from build123d import *

# Parameters (mm, degrees)
SKETCH_1_W      = 450
SKETCH_1_H      = 390
SKETCH_1_R      = 157.5
SKETCH_1_R_2    = 6
SKETCH_1_R_3    = 20
EXTRUDE_1_DEPTH = 24


with BuildPart() as part:
    # 草图1 → 凸台-拉伸1 (new body)
    with BuildSketch(Plane.XY):
        Rectangle(SKETCH_1_W, SKETCH_1_H)
        with Locations((-45, 0)):
            Circle(SKETCH_1_R, mode=Mode.SUBTRACT)
        with Locations((-205, 85)):
            Circle(SKETCH_1_R_2, mode=Mode.SUBTRACT)
        with Locations(Location((-205, -85, 0), (0, 0, 180))):
            Circle(SKETCH_1_R_2, mode=Mode.SUBTRACT)
        with Locations((40, 160)):
            Circle(SKETCH_1_R_2, mode=Mode.SUBTRACT)
        with Locations(Location((-130, 160, 0), (0, 0, 180))):
            Circle(SKETCH_1_R_2, mode=Mode.SUBTRACT)
        with Locations((115, -85)):
            Circle(SKETCH_1_R_2, mode=Mode.SUBTRACT)
        with Locations(Location((115, 85, 0), (0, 0, 180))):
            Circle(SKETCH_1_R_2, mode=Mode.SUBTRACT)
        with Locations((-130, -160)):
            Circle(SKETCH_1_R_2, mode=Mode.SUBTRACT)
        with Locations(Location((40, -160, 0), (0, 0, 180))):
            Circle(SKETCH_1_R_2, mode=Mode.SUBTRACT)
        with Locations((165, 135)):
            Circle(SKETCH_1_R_3, mode=Mode.SUBTRACT)
    extrude(amount=EXTRUDE_1_DEPTH)


solid = part.part
Input: part model. Units: mm. Frame: model coordinates. Give positions to 0.01 mm unless a question says otherwise; leave off trailing zeros. Loops run counter-clockwise (first coordinate to the right, second up) from the corner with the lowest first, then second, coordinate; pieces in that order, holes last. Notation, with made-up numbers: (-36, 2) -> (1, 2) arc R5 ccw to (1, 9) -> close; hole circle Ø8 at (-25.75, 35.5). An arc over 180 degrees is marked (long way). Answer as a JSON object with one key per item and string values. Group by question number.
Item 1: Cut plane C-C, the plane y = 47.5. Return the cut outline in (x, z).
Item 2: Cut plane B-B, the plane x = -45. Return the cut outline in (y, z).
Item 3: Pin query (flat end, axial travel): P1, Ø14, axis at x = 115, y = -85, coming from the -Z side. Return the tip coordinate at first contact, or that it passes through.
Item 4: Pull-direction query (X, two-part tool) for faces 1 (the cylindrical face through (-134.76, -163.65, 11.83)), 2 (the flat face through (-3, 195, 12)), 3 (the flat face through (-225, -3, 12)); classes: released by +X, released by -X, zero draft, split by the parting line, or undercut.
Item 5: Cut plane D-D, the plane x = -130. Return the cut outline in (y, z), and give its area (3 significant figures).
Item 6: Line query: probe 1 along Y at (x, z) = (115, 6.25); probe 2 along Y at (x, z) = (-42.5, 14.5); probe 3 along Y at (x, z) = (-130, 5). Output: solid intervals per line, ascending.
Item 7: Cut plane A-A, the plane z = 8.25. State how many separate pieces and enclosed holes the cut face has, and give its area (3 significant figures).
Checks:
{
 "1": {"outline": "(-225, 0) -> (-195.17, 0) -> (-195.17, 24) -> (-225, 24) -> close; (105.17, 0) -> (225, 0) -> (225, 24) -> (105.17, 24) -> close"},
 "2": {"outline": "(-195, 0) -> (-157.5, 0) -> (-157.5, 24) -> (-195, 24) -> close; (157.5, 0) -> (195, 0) -> (195, 24) -> (157.5, 24) -> close"},
 "3": {"P1": "stops at z = 0"},
 "4": {"face 1": "undercut", "face 2": "zero draft", "face 3": "released by -X"},
 "5": {"outline": "(-195, 0) -> (-166, 0) -> (-166, 24) -> (-195, 24) -> close; (-154, 0) -> (-132.59, 0) -> (-132.59, 24) -> (-154, 24) -> close; (132.59, 0) -> (154, 0) -> (154, 24) -> (132.59, 24) -> close; (166, 0) -> (195, 0) -> (195, 24) -> (166, 24) -> close", "area": "2,420 mm²"},
 "6": {"probe 1": "y = -195 to -91, -79 to 79, 91 to 195", "probe 2": "y = -195 to -157.48, 157.48 to 195", "probe 3": "y = -195 to -166, -154 to -132.59, 132.59 to 154, 166 to 195"},
 "7": {"separate pieces": "1", "enclosed holes": "10", "area": "95,400 mm²"}
}
